Read the model definition and answer for the solid it produces. Units are mm, in the model's axes. A direction names the side the tool comes from. Give positions to 0.01 mm unless a question says otherwise; leave off trailing zeros. Loops run counter-clockwise (first coordinate to the right, second up) from the corner with the lowest first, then second, coordinate; pieces in that order, holes last. Notation, with made-up numbers: (-14, 30) - (28, 30) arc R20 ccw to (28, 49) - close; hole circle Ø3 at (-4, -16.75). An arc over 180 degrees is marked (long way). Put each result on its own line as item: value. Start each with the question number.
1. Given pin 1 Ø1 at (x, z) = (23.5, 22.5) entering from +Y; pin 2 Ø0.6 at (y, z) = (79, 22) entering from -X; pin 3 Ø12 at (y, z) = (70.5, 26.5) entering from +X, each flat-ended and moving along its own axis, determine where each tip first touches the part or whether it passes through.
2. For faces 1 (the cylindrical face through (15, 79, 17)), 2 (the cylindrical face through (15.465, 7.182, 25.399)), 3 (the flat face through (14, 1, 15)), determine the directions among +Z, -Z, +X, -X, +Y, -Y from which every point of the face is accessible in a straight line to the end or side of a thin tool.
3. A cutting plane is placed at D-D, the plane y = 27.5. Determine the outline of the cut face in (x, z), plus the area to 3 significant figures.
4. A cutting plane is placed at C-C, the plane x = 23.5. Determine the outline of the cut face in (y, z).
5. A cutting plane is placed at A-A, the plane y = 51. Determine the outline of the cut face in (x, z).
6. A cutting plane is placed at B-B, the plane x = 15. Count the separate pieces of the cut face and the enclosed holes in it, plus the area to 3 significant figures.
7. For a pull along Y with two mould halves and no side action, classify faces 4 (the flat face through (11, 39, 4)), 5 (the flat face through (0, 37, 3)), 6 (the flat face through (15, 0, 15)) as released by +Y, released by -Y, zero draft, split by the parting line, or undercut.
8. Consider L1, parallel to Z at x = 15, y = 79.15; L2, parallel to Y at x = 17.25, z = 9.3; L3, parallel to Z at x = 7.75, y = 11. Determine where each line is inside the solid, lowest interval first. Write a range as from..to.
```python
from build123d import *

# Parameters (mm, degrees)
BOX_W           = 30
BOX_H           = 80
BOX_DEPTH       = 30
SKETCH_W        = 75
SKETCH_H        = 21
POCKET_DEPTH    = 10
SKETCH001_W     = 76
SKETCH001_H     = 22
POCKET001_DEPTH = 18
POCKET002_DEPTH = 78
SKETCH003_W     = 6
SKETCH003_H     = 8
PAD_DEPTH       = 5
FILLET_R        = 2
POCKET003_DEPTH = 3
FILLET001_R     = 0.2
SKETCH005_R     = 1.5
POCKET004_DEPTH = 19
SKETCH006_R     = 1.5
SKETCH006_R_2   = 2.5
POCKET005_DEPTH = 5
PAD001_DEPTH    = 13
SKETCH008_R     = 1.5
POCKET006_DEPTH = 8
SKETCH009_W     = 75
SKETCH009_H     = 25
POCKET007_DEPTH = 10


with BuildPart() as part:
    # Box → Box (join)
    with BuildSketch(Plane.XY):
        with Locations((15, 40)):
            Rectangle(BOX_W, BOX_H)
    extrude(amount=BOX_DEPTH)

    # Sketch (on Face2 of Box) → Pocket (cut)
    with BuildSketch(Plane.YZ.offset(30)):
        with Locations((42.5, 15)):
            Rectangle(SKETCH_W, SKETCH_H)
    extrude(amount=-POCKET_DEPTH, mode=Mode.SUBTRACT)

    # Sketch001 → Pocket001 (cut)
    with BuildSketch(Plane.YZ):
        with Locations((40, 15)):
            Rectangle(SKETCH001_W, SKETCH001_H)
    extrude(amount=POCKET001_DEPTH, mode=Mode.SUBTRACT)

    # Sketch002 (on Face5 of Pocket001) → Pocket002 (cut)
    with BuildSketch(Plane(origin=(0, 80, 0), x_dir=(-1, 0, 0), z_dir=(0, 1, 0))):
        Polygon((-4, 28), (-2, 28), (0, 26), (5, 26), (5, 4), (0, 4), (-2, 2), (-4, 2), align=None)
    extrude(amount=-POCKET002_DEPTH, mode=Mode.SUBTRACT)

    # Sketch003 → Pad (join)
    with BuildSketch(Plane.YZ.offset(18)):
        with Locations((51, 22)):
            Rectangle(SKETCH003_W, SKETCH003_H)
        with Locations((51, 8)):
            Rectangle(SKETCH003_W, SKETCH003_H)
        with Locations((3.611342, 22)):
            Rectangle(SKETCH003_W, SKETCH003_H)
        with Locations((4, 8)):
            Rectangle(SKETCH003_W, SKETCH003_H)
    extrude(amount=-PAD_DEPTH)

    # Fillet
    fillet_edges = [part.edges().sort_by_distance(p)[0] for p in [
        (15.5, 2, 18),
        (15.5, 2, 12),
        (15.5, 7, 12),
        (15.5, 6.611342, 18),
        (15.5, 48, 12),
        (15.5, 54, 12),
        (15.5, 48, 4),
        (15.5, 54, 4),
        (15.5, 54, 18),
        (15.5, 48, 18),
        (15.5, 48, 26),
        (15.5, 54, 26),
        (15.5, 7, 4),
        (15.5, 6.611342, 26),
    ]]
    fillet(fillet_edges, radius=FILLET_R)

    # Sketch004 (on Face46 of Fillet) → Pocket003 (cut)
    with BuildSketch(Plane.XZ):
        with BuildLine():
            ThreePointArc((14, 18.5), (10, 22.5), (6, 18.5))
            Line((6, 18.5), (6, 11.5))
            ThreePointArc((6, 11.5), (10, 7.5), (14, 11.5))
            Line((14, 11.5), (14, 18.5))
        make_face()
    extrude(amount=-POCKET003_DEPTH, mode=Mode.SUBTRACT)

    # Fillet001
    fillet001_edges = [part.edges().sort_by_distance(p)[0] for p in [
        (13, 3, 19.438901),
        (13.5, 3, 17.732051),
        (13.5, 3, 12.267949),
        (13, 3, 10.561099),
    ]]
    fillet(fillet001_edges, radius=FILLET001_R)

    # Sketch005 → Pocket004 (cut)
    with BuildSketch(Plane.YZ):
        with Locations((4, 9.3)):
            Circle(SKETCH005_R)
        with Locations((4, 20.7)):
            Circle(SKETCH005_R)
        with Locations((51, 9.3)):
            Circle(SKETCH005_R)
        with Locations((51, 20.7)):
            Circle(SKETCH005_R)
    extrude(amount=POCKET004_DEPTH, mode=Mode.SUBTRACT)

    # Sketch006 (on Face58 of Pocket004) → Pocket005 (cut)
    with BuildSketch(Plane(origin=(0, 80, 0), x_dir=(-1, 0, 0), z_dir=(0, 1, 0))):
        with Locations((-15, 13)):
            Circle(SKETCH006_R)
        with Locations((-15, 7)):
            Circle(SKETCH006_R_2)
        with BuildLine():
            ThreePointArc((-13, 23), (-15, 25), (-17, 23))
            Line((-17, 23), (-17, 19))
            ThreePointArc((-17, 19), (-15, 17), (-13, 19))
            Line((-13, 19), (-13, 23))
        make_face()
    extrude(amount=-POCKET005_DEPTH, mode=Mode.SUBTRACT)

    # Sketch007 → Pad001 (join, symmetric)
    with BuildSketch(Plane.XY.offset(15)):
        with BuildLine():
            Line((4, 80), (10, 80))
            ThreePointArc((4, 74), (8.242641, 75.757359), (10, 80))
            Line((4, 80), (4, 74))
        make_face()
    extrude(amount=PAD001_DEPTH, both=True)

    # Sketch008 → Pocket006 (cut)
    with BuildSketch(Plane.YZ):
        with Locations((77, 15)):
            Circle(SKETCH008_R)
    extrude(amount=POCKET006_DEPTH, mode=Mode.SUBTRACT)

    # Sketch009 (on Face49 of Pocket006) → Pocket007 (cut)
    with BuildSketch(Plane.YZ.offset(30)):
        with Locations((42.5, 32.5)):
            Rectangle(SKETCH009_W, SKETCH009_H)
    extrude(amount=-POCKET007_DEPTH, mode=Mode.SUBTRACT)


solid = part.part
```
Return value:
1. pin 1: stops at y = 5
1. pin 2: stops at x = 4
1. pin 3: stops at x = 20
2. face 1: +Y
2. face 2: -X
2. face 3: -Y
3. outline: (0, 0) - (30, 0) - (30, 4.5) - (20, 4.5) - (20, 30) - (0, 30) - (0, 26) - (2, 28) - (4, 28) - (4, 26) - (18, 26) - (18, 4) - (4, 4) - (4, 2) - (2, 2) - (0, 4) - close
3. area: 237 mm2
4. outline: (0, 0) - (80, 0) - (80, 4.5) - (5, 4.5) - (5, 30) - (0, 30) - close
5. outline: (0, 0) - (30, 0) - (30, 4.5) - (20, 4.5) - (20, 30) - (0, 30) - (0, 26) - (2, 28) - (4, 28) - (4, 26) - (13, 26) - (13, 22.2) - (19, 22.2) - (19, 19.2) - (13, 19.2) - (13, 18) - (18, 18) - (18, 12) - (13, 12) - (13, 10.8) - (19, 10.8) - (19, 7.8) - (13, 7.8) - (13, 4) - (4, 4) - (4, 2) - (2, 2) - (0, 4) - close
6. separate pieces: 3
6. enclosed holes: 4
6. area: 842 mm2
7. face 4: undercut
7. face 5: zero draft
7. face 6: released by -Y
8. L1: z = 0..4.5, 9.5..11.5, 14.5..17, 25..30
8. L2: y = 0..2.5, 5.5..7, 48..49.5, 52.5..54, 78..80
8. L3: z = 0..4, 26..30
